Geometry check sheet. Reference: the model listing, model coordinates, mm. A direction names the side the tool comes from. Round coordinates to 2 decimals unless told otherwise and drop trailing zeros. Order: outer loops, then holes, each group sorted by start corner. A loop starts at its lowest first (then second) coordinate and runs counter-clockwise, first axis right, second up. Notation, with made-up numbers: (52, 77) - (109, 77) arc R19 cw to (109, 89) - close; hole circle Ø5 at (70.25, 14). An arc over 180 degrees is marked (long way). Answer as CSV lines item,"result". Start each with the question number.
```python
from build123d import *

# Parameters (mm, degrees)
BOSS_EXTRUDE1_DEPTH   = 80
SKETCH2_R             = 26
CUT_EXTRUDE1_DEPTH    = 0.6
FILLET1_R             = 0.6
SKETCH3_R             = 23
CUT_EXTRUDE2_DEPTH    = 4.4
M6X1_0_TAPPED_HOLE1_D = 5
M6X1_0_TAPPED_HOLE2_D = 5


with BuildPart() as part:
    # Sketch1 → Boss-Extrude1 (new body)
    with BuildSketch(Plane.XY):
        Polygon((0, 35), (20, 35), (20, -35), (0, -35), (0, -40), (25, -40), (25, 40), (0, 40), align=None)
    extrude(amount=BOSS_EXTRUDE1_DEPTH)

    # Sketch2 → Cut-Extrude1 (cut)
    with BuildSketch(Plane.ZY.offset(-20)):
        with Locations(Location((40, 0, 0), (0, 0, 270))):
            Circle(SKETCH2_R)
    extrude(amount=-CUT_EXTRUDE1_DEPTH, mode=Mode.SUBTRACT)

    # Fillet1
    fillet1_edges = [part.edges().sort_by_distance(p)[0] for p in [
        (20.6, 26, 40),
    ]]
    fillet(fillet1_edges, radius=FILLET1_R - 0.0001)  # a hair under: the kernel refuses the full size

    # Sketch3 → Cut-Extrude2 (cut)
    with BuildSketch(Plane.ZY.offset(-20.6)):
        with Locations(Location((40, 0, 0), (0, 0, 270))):
            Circle(SKETCH3_R)
    extrude(amount=-CUT_EXTRUDE2_DEPTH, mode=Mode.SUBTRACT)

    # M6x1.0 Tapped Hole1 (through all)
    with Locations(Plane(origin=(0, 40, 0), x_dir=(1, 0, 0), z_dir=(0, 1, 0))):
        with Locations((10, -17.4), (10, -62.6)):
            Hole(M6X1_0_TAPPED_HOLE1_D / 2)

    # M6x1.0 Tapped Hole2 (through all)
    with Locations(Plane(origin=(25, 0, 0), x_dir=(0, 0, -1), z_dir=(1, 0, 0))):
        with Locations((-72, 27.5), (-8, 27.5), (-8, -27.5), (-72, -27.5)):
            Hole(M6X1_0_TAPPED_HOLE2_D / 2)


solid = part.part
```
1. Access from +Z, -Z, +X, -X, +Y, -Y to the whole of each face (thin tool, end or side, straight path). Record for faces 1 (the face through (20, 0, 13)), 2 (the face through (20.6, 4, 63)), 3 (the face through (11.84, -37.53, 15.71)).
2. Section check C-C on y = -27.5. Record the boundary of the cut face in (x, z).
3. Draft check along Z on faces 4 (the face through (10, -35, 39)), 5 (the face through (21, 3, 0)), 6 (the face through (22.47, -25.39, 9.34)), 7 (the face through (21, 3, 80)). Enter one of: released by +Z, released by -Z, zero draft, split by the parting line, or undercut.
4. Go/stop test with a flat-tipped pin: pin 1 Ø3 at (y, z) = (29, 61.5) entering from -X. Record where the tip stops, or that it passes through.
5. Section check D-D on x = 10. Record the boundary of the cut face in (y, z).
6. Thickness scan on probe 1 along Z at (x, y) = (10, -36.6); probe 2 along X at (y, z) = (-38.05, 62.6); probe 3 along Y at (x, z) = (5.25, 24). Record the ranges inside material, lowest first.
7. Section check B-B on z = 72. Record the boundary of the cut face in (x, y).
8. Section check A-A on x = 17.5. Record the boundary of the cut face in (y, z), plus the area to 3 significant figures.
Numbers:
1,face 1,"+Z, -Z, -X"
1,face 2,"-X"
1,face 3,"+Y, -Y"
2,outline,"(20, 0) - (25, 0) - (25, 5.5) - (20, 5.5) - close; (20, 10.5) - (25, 10.5) - (25, 69.5) - (20, 69.5) - close; (20, 74.5) - (25, 74.5) - (25, 80) - (20, 80) - close"
3,face 4,"zero draft"
3,face 5,"released by -Z"
3,face 6,"undercut"
3,face 7,"released by +Z"
4,pin 1,"stops at x = 20"
5,outline,"(-40, 0) - (-35, 0) - (-35, 14.9) - (-40, 14.9) - close; (-40, 19.9) - (-35, 19.9) - (-35, 60.1) - (-40, 60.1) - close; (-40, 65.1) - (-35, 65.1) - (-35, 80) - (-40, 80) - close; (35, 0) - (40, 0) - (40, 14.9) - (35, 14.9) - close; (35, 19.9) - (40, 19.9) - (40, 60.1) - (35, 60.1) - close; (35, 65.1) - (40, 65.1) - (40, 80) - (35, 80) - close"
6,probe 1,"z = 0 to 14.9, 19.9 to 60.1, 65.1 to 80"
6,probe 2,"x = 0 to 7.5, 12.5 to 25"
6,probe 3,"y = -40 to -35, 35 to 40"
7,outline,"(0, -40) - (25, -40) - (25, -30) - (20, -30) - (20, -35) - (0, -35) - close; (0, 35) - (20, 35) - (20, 30) - (25, 30) - (25, 40) - (0, 40) - close; (20, -25) - (25, -25) - (25, 25) - (20, 25) - close"
8,outline,"(-40, 0) - (-35, 0) - (-35, 80) - (-40, 80) - close; (35, 0) - (40, 0) - (40, 80) - (35, 80) - close"
8,area,"800 mm2"
